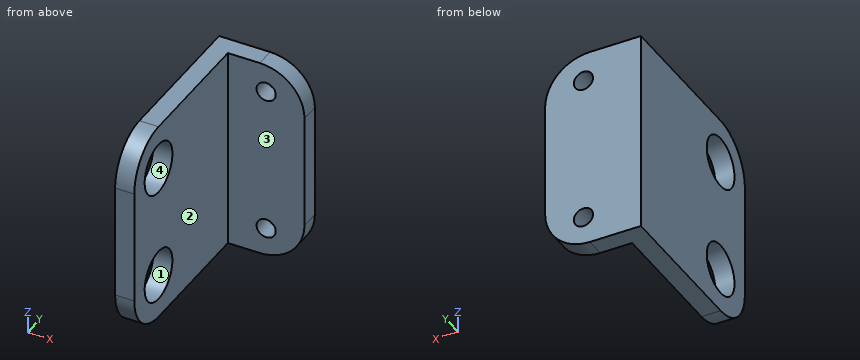
Autodesk Inventor part; units mm, degrees
ref_plane "YZ Plane" through (0, 0, 0) normal (1, 0, 0) x (0, 1, 0)
ref_plane "XZ Plane" through (0, 0, 0) normal (0, 1, 0) x (-1, 0, 0)
ref_plane "XY Plane" through (0, 0, 0) normal (0, 0, 1) x (1, 0, 0)
sketch "Sketch1" plane through (0, 0, 0) normal (0, 0, 1) x (1, 0, 0)
  line L0 (0, 0) -> (0, 30)
  line L1 (0, 30) -> (15, 30)
  line L2 (15, 30) -> (15, 27)
  line L3 (15, 27) -> (3, 27)
  line L4 (3, 27) -> (3, 0)
  line L5 (3, 0) -> (0, 0)
  dimension "d0" = 30
  dimension "d1" = 12
  dimension "d2" = 3
  dimension "d3" = 3
extrude "Extrusion1" add sketch "Sketch1" along normal blind 32
fillet "Fillet1" radius 7 2 edges at (1.5, 0, 32) (1.5, 0, 0)
sketch "Sketch2" plane through (3, 27, 32) normal (1, 0, 0) x (0, 0, -1)
  line L0 (0, -20) -> (0, 0)
  line L1 (32, 3) -> (0, 3)
  point P0 (32, -27)
  point P1 (7, -20)
  point P2 (25, -20)
  dimension "d7" = 18
  dimension "d8" = 7
  dimension "d9" = 23
  dimension "d10" = 23
hole "Hole1" at (3, 7, 25) at (3, 7, 7) direction (-1, 0, 0) diameter 8 end through all
sketch "Sketch3" plane through (0, 30, 0) normal (0, 1, 0) x (1, 0, 0)
  line L0 (15, 0) -> (0, 0)
  line L1 (0, 0) -> (0, -32)
  point P0 (9, -27.5)
  point P1 (9, -4.5)
  dimension "d18" = 23
  dimension "d19" = 4.5
  dimension "d20" = 9
  dimension "d21" = 9
hole "Hole2" at (9, 30, 27.5) at (9, 30, 4.5) direction (0, -1, 0) diameter 3 end through all
fillet "Fillet2" radius 7 2 edges at (15, 28.5, 0) (15, 28.5, 32)
properties part number "HUDSON-1-76"
Geometry: final body of the model. Coordinates: model frame, mm. Face numbers are marked on the shaded views. Coordinates: 2 decimals unless noted, no trailing zeros. Order: outer loops, then holes, each group sorted by start corner. A loop starts at its lowest first (then second) coordinate and runs counter-clockwise, first axis right, second up.
1) Section B-B (z = 25.5). Return loops of the section in (x, y), then the cut area to 3 significant figures.
Result sheet:
outline: (0, 0.02) - (3, 0.02) - (3, 3.03) - (0, 3.03) - close; (0, 10.97) - (3, 10.97) - (3, 27) - (14.98, 27) - (14.98, 30) - (0, 30) - close
area: 102 mm2
2) Ray query, probe 1 along Z at (x, y) = (1.1, 7); probe 2 along Z at (x, y) = (9, 28.65); probe 3 along X at (y, z) = (11, 20). Return the intervals inside material, ascending.
Result sheet:
probe 1: z = 0 to 3, 11 to 21, 29 to 32
probe 2: z = 0.07 to 3, 6 to 26, 29 to 31.93
probe 3: x = 0 to 3
3) Draft query along Y for the marked faces 1, 2, 3 and 4. Return one class per face: released by +Y, released by -Y, zero draft, split by the parting line, or undercut.
Result sheet:
face 1: undercut
face 2: zero draft
face 3: released by -Y
face 4: undercut
4) Section A-A (y = 27.5). Return loops of the section in (x, z), then the cut area to 3 significant figures.
Result sheet:
outline: (0, 0) - (8, 0) arc R7 ccw to (15, 7) - (15, 25) arc R7 ccw to (8, 32) - (0, 32) - close; hole circle Ø3 at (9, 4.5); hole circle Ø3 at (9, 27.5)
area: 445 mm2
5) Section C-C (y = 7.5). Return loops of the section in (x, z), then the cut area to 3 significant figures.
Result sheet:
outline: (0, 0) - (3, 0) - (3, 3.03) - (0, 3.03) - close; (0, 10.97) - (3, 10.97) - (3, 21.03) - (0, 21.03) - close; (0, 28.97) - (3, 28.97) - (3, 32) - (0, 32) - close
area: 48.4 mm2
6) First-contact query: P1, Ø5, axis at y = 7, z = 25, coming from the +X side; P2, Ø5, axis at x = 9, z = 4.5, coming from the -Y side; P3, Ø8, axis at y = 13.5, z = 10, coming from the +X side. Flat tips, straight axial feed; report the tip coordinate or a pass-through.
Result sheet:
P1: passes through
P2: stops at y = 27
P3: stops at x = 3
7) Section D-D (x = 9). Return loops of the section in (y, z), then the cut area to 3 significant figures.
Result sheet:
outline: (27, 0.07) - (30, 0.07) - (30, 3) - (27, 3) - close; (27, 6) - (30, 6) - (30, 26) - (27, 26) - close; (27, 29) - (30, 29) - (30, 31.93) - (27, 31.93) - close
area: 77.6 mm2
